The model under review builds one solid part; all positions refer to its coordinate system, in mm. A direction names the side the tool comes from. Round coordinates to 2 decimals unless told otherwise and drop trailing zeros. Order: outer loops, then holes, each group sorted by start corner. A loop starts at its lowest first (then second) coordinate and runs counter-clockwise, first axis right, second up.
```python
from build123d import *

# Parameters (mm, degrees)
F0_R     = 76.420931
F0_R_2   = 70.062958
F1_DEPTH = 27.94
F3_DEPTH = 51.562


with BuildPart() as f1:
    # F0 (on Top) → F1 (new body)
    with BuildSketch(Plane.XY):
        Circle(F0_R)
        Circle(F0_R_2, mode=Mode.SUBTRACT)
    extrude(amount=F1_DEPTH)

    # F2 (on Front) → F3 (join)
    with BuildSketch(Plane.XZ):
        Polygon((-38.800031, 57.597559), (-57.838555, 26.750332), (53.81551, 27.955303), (33.257172, 57.597559), (12.531687, 27.955303), (-16.329287, 27.955303), align=None)
    extrude(amount=F3_DEPTH)


solid = f1.part
```
(1) For faces 1 (the flat face through (43.68, -25.42, 42.57)), 2 (the flat face through (-2, -25, 27.955)), list the 3-axis set-ups (+Z, -Z, +X, -X, +Y, -Y) from which the entire face can be reached by the end or side of a thin tool; tool diameter is ignored.
Data:
face 1: +Z, +X, +Y, -Y
face 2: +Z, +Y, -Y
(2) Insertion check: pin 1 (24.5 mm diameter, centred on x = 13.5, z = 44, fed in from +Y); pin 2 (8.5 mm diameter, centred on x = 5.5, y = -22, fed in from +Z); pin 3 (12 mm diameter, centred on y = 58.5, z = 11.5, fed in from +X). Each pin has a flat end and moves straight along its axis. Give the tip position at first contact, or say it passes through.
Data:
pin 1: stops at y = 0
pin 2: stops at z = 27.96
pin 3: stops at x = 55.53
(3) Consider section B-B (x = 24.5). Write out the cut boundary in (y, z), and give its area (3 significant figures).
Data:
outline: (-72.39, 0) - (-65.64, 0) - (-65.64, 27.94) - (-72.39, 27.94) - close; (-51.56, 27.64) - (0, 27.64) - (0, 45.07) - (-51.56, 45.07) - close; (65.64, 0) - (72.39, 0) - (72.39, 27.94) - (65.64, 27.94) - close
area: 1,280 mm2
(4) Draft analysis for pull direction X (two halves, no side actions). For faces 3 (the flat face through (-27.41, -25.42, 42.57)), 4 (the flat face through (23.04, -25.42, 42.984)), 5 (the flat face through (34, -62, 0)), 6 (the cylindrical face through (-60.645, -46.501, 13.774)), state which applies: pulls with the +X half, pulls with the -X half, needs draft (parallel to the pull), parting line crosses it, or undercut.
Data:
face 3: undercut
face 4: undercut
face 5: needs draft
face 6: parting line crosses it
(5) Consider section C-C (z = 49). Write out the cut boundary in (x, y), and give its area (3 significant figures).
Data:
outline: (-44.11, -51.56) - (-32.28, -51.56) - (-32.28, 0) - (-44.11, 0) - close; (27.25, -51.56) - (39.22, -51.56) - (39.22, 0) - (27.25, 0) - close
area: 1,230 mm2
(6) To check wall thickness, follow probe 1 along Y at (x, z) = (0, 17); probe 2 along Z at (x, y) = (-36, 60.5). State the ranges of each line that lie inside material, in increasing order.
Data:
probe 1: y = -76.42 to -70.06, 70.06 to 76.42
probe 2: z = 0 to 27.94
(7) Consider section D-D (y = -4.5). Write out the cut boundary in (x, z), and give its area (3 significant figures).
Data:
outline: (-76.29, 0) - (-69.92, 0) - (-69.92, 27.94) - (-76.29, 27.94) - close; (-57.84, 26.75) - (53.82, 27.96) - (33.26, 57.6) - (12.53, 27.96) - (-16.33, 27.96) - (-38.8, 57.6) - close; (69.92, 0) - (76.29, 0) - (76.29, 27.94) - (69.92, 27.94) - close
area: 1,640 mm2
(8) Consider section A-A (y = 33). Write out the cut boundary in (x, z), and give its area (3 significant figures).
Data:
outline: (-68.93, 0) - (-61.8, 0) - (-61.8, 27.94) - (-68.93, 27.94) - close; (61.8, 0) - (68.93, 0) - (68.93, 27.94) - (61.8, 27.94) - close
area: 398 mm2
